```python
from build123d import *

# Parameters (mm, degrees)
BOSS_EXTRUDE1_DEPTH = 1.5
SKETCH2_R           = 1
CUT_EXTRUDE1_DEPTH  = 13.678722333
CHAMFER1_SIZE       = 0.1
FILLET1_R           = 0.2


with BuildPart() as part:
    # Sketch1 → Boss-Extrude1 (new body)
    with BuildSketch(Plane(origin=(0, 0, 0), x_dir=(1, 0, 0), z_dir=(0, 1, 0))):
        with BuildLine():
            Line((7.5, -0.75), (7.5, -1.5))
            Line((7.5, -1.5), (11.5, -1.5))
            ThreePointArc((11.5, -1.5), (12.207106781, -1.207106781), (12.5, -0.5))
            Line((12.5, -0.5), (12.5, 0.5))
            ThreePointArc((12.5, 0.5), (12.207106781, 1.207106781), (11.5, 1.5))
            Line((11.5, 1.5), (7.5, 1.5))
            Line((7.5, 1.5), (7.5, 0.75))
            Line((7.5, 0.75), (-7.5, 0.75))
            Line((-7.5, 0.75), (-7.5, 1.5))
            Line((-7.5, 1.5), (-11.5, 1.5))
            ThreePointArc((-11.5, 1.5), (-12.207106781, 1.207106781), (-12.5, 0.5))
            Line((-12.5, 0.5), (-12.5, -0.5))
            ThreePointArc((-12.5, -0.5), (-12.207106781, -1.207106781), (-11.5, -1.5))
            Line((-11.5, -1.5), (-7.5, -1.5))
            Line((-7.5, -1.5), (-7.5, -0.75))
            Line((-7.5, -0.75), (7.5, -0.75))
        make_face()
    extrude(amount=BOSS_EXTRUDE1_DEPTH)

    # Sketch2 → Cut-Extrude1 (cut, through all)
    with BuildSketch(Plane(origin=(0, 1.5, 0), x_dir=(1, 0, 0), z_dir=(0, 1, 0))):
        with Locations(Location((-11, 0, 0), (0, 0, 270))):
            Circle(SKETCH2_R)
        with Locations(Location((11, 0, 0), (0, 0, 270))):
            Circle(SKETCH2_R)
    extrude(amount=-CUT_EXTRUDE1_DEPTH, mode=Mode.SUBTRACT)

    # Chamfer1
    chamfer1_edges = [part.edges().sort_by_distance(p)[0] for p in [
        (-11, 0, -1),
        (-11, 1.5, -1),
        (11, 0, -1),
        (11, 1.5, -1),
    ]]
    chamfer(chamfer1_edges, length=CHAMFER1_SIZE)

    # Fillet1
    fillet1_edges = [part.edges().sort_by_distance(p)[0] for p in [
        (7.5, 0, 1.125),
        (7.5, 0, -1.125),
        (0, 0, 0.75),
        (12.5, 1.5, 0),
        (7.5, 1.5, 1.125),
        (0, 1.5, 0.75),
        (-12.5, 1.5, 0),
        (-7.5, 1.5, -1.125),
        (7.5, 1.5, -1.125),
        (-7.5, 0.75, -1.5),
        (-9.5, 1.5, -1.5),
        (-9.5, 0, -1.5),
        (7.5, 0.75, -0.75),
        (0, 1.5, -0.75),
        (0, 0, -0.75),
        (9.5, 1.5, -1.5),
        (7.5, 0.75, -1.5),
        (9.5, 0, -1.5),
        (-9.5, 1.5, 1.5),
        (-7.5, 0.75, 1.5),
        (-9.5, 0, 1.5),
        (7.5, 0.75, 1.5),
        (9.5, 1.5, 1.5),
        (9.5, 0, 1.5),
        (12.207106781, 0, -1.207106781),
        (12.5, 0, 0),
        (12.207106781, 0, 1.207106781),
        (12.207106781, 1.5, -1.207106781),
        (12.207106781, 1.5, 1.207106781),
        (-12.207106781, 0, 1.207106781),
        (-12.5, 0, 0),
        (-12.207106781, 0, -1.207106781),
        (-12.207106781, 1.5, 1.207106781),
        (-12.207106781, 1.5, -1.207106781),
    ]]
    fillet(fillet1_edges, radius=FILLET1_R)


solid = part.part
```
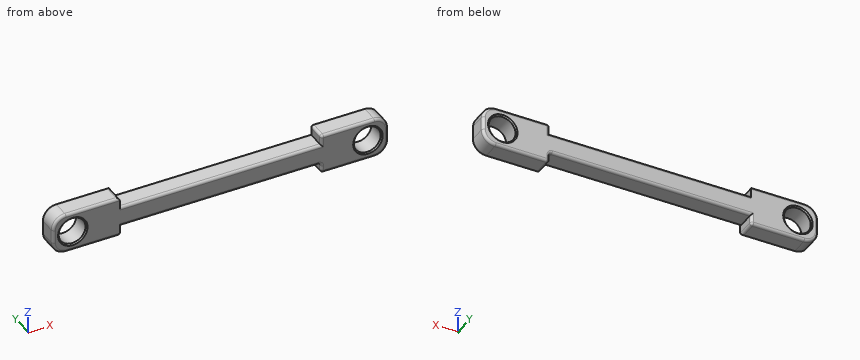
The model under review builds one solid part; all positions refer to its coordinate system, in mm. Round coordinates to 2 decimals unless told otherwise and drop trailing zeros. Loops run counter-clockwise (first coordinate to the right, second up) from the corner with the lowest first, then second, coordinate; pieces in that order, holes last.
1) Consider section B-B on z = 0. State the section outline as (x, y) points.
Values follow:
outline: (-12.5, 0.2) arc R0.2 ccw to (-12.3, 0) - (-12.1, 0) - (-12, 0.1) - (-12, 1.4) - (-12.1, 1.5) - (-12.3, 1.5) arc R0.2 ccw to (-12.5, 1.3) - close; (-10, 0.1) - (-9.9, 0) - (9.9, 0) - (10, 0.1) - (10, 1.4) - (9.9, 1.5) - (-9.9, 1.5) - (-10, 1.4) - close; (12, 0.1) - (12.1, 0) - (12.3, 0) arc R0.2 ccw to (12.5, 0.2) - (12.5, 1.3) arc R0.2 ccw to (12.3, 1.5) - (12.1, 1.5) - (12, 1.4) - close
2) Consider section A-A on x = -11. State the section outline as (y, z) points.
Values follow:
outline: (0, -1.3) arc R0.2 ccw to (0.2, -1.5) - (1.3, -1.5) arc R0.2 ccw to (1.5, -1.3) - (1.5, -1.1) - (1.4, -1) - (0.1, -1) - (0, -1.1) - close; (0, 1.1) - (0.1, 1) - (1.4, 1) - (1.5, 1.1) - (1.5, 1.3) arc R0.2 ccw to (1.3, 1.5) - (0.2, 1.5) arc R0.2 ccw to (0, 1.3) - close
3) Clearance check with flat-ended pins moving along their axes: P1, Ø0.6, axis at x = 1.5, y = 1, coming from the +Z side; P2, Ø0.8, axis at y = 0.5, z = -1, coming from the +X side (3 decimals). State where each tip first meets the part, or that it passes through.
Values follow:
P1: stops at z = 0.75
P2: stops at x = 12.495
4) Wall thickness on line 1 along X through (y, z) = (0.6, -0.1); line 2 along X through (y, z) = (1.3, 0.8); line 3 along X through (y, z) = (1.45, -0.1): over which ranges is each line inside the solid? List them lowest first.
Values follow:
line 1: x = -12.5 to -11.99, -10.01 to 10.01, 11.99 to 12.5
line 2: x = -12.45 to -11.6, -10.4 to -7.5, 7.5 to 10.4, 11.6 to 12.45
line 3: x = -12.43 to -12.05, -9.95 to 9.95, 12.05 to 12.43
